from build123d import *

# Parameters (mm, degrees)
F1_DEPTH  = 12
F2_R      = 8
F3_DEPTH  = 12
F4_R      = 26
F5_DEPTH  = 46
F6_R      = 15
F7_DEPTH  = 12
F8_R      = 10
F9_DEPTH  = 34
F10_R     = 30
F10_R_2   = 26
F11_DEPTH = 12
F13_DEPTH = 46
F14_W     = 44.7685575615
F14_H     = 8
F15_DEPTH = 46
F17_DEPTH = 25


with BuildPart() as f1:
    # F0 (on Top) → F1 (new body)
    with BuildSketch(Plane.XY):
        with BuildLine():
            ThreePointArc((-54.3153104275, 3.1455838755), (-49.6290189265, -8.1681246235), (-38.3153104275, -12.8544161245))
            Line((-38.3153104275, -12.8544161245), (57.6846895725, -12.8544161245))
            ThreePointArc((57.6846895725, -12.8544161245), (68.9983980715, -8.1681246235), (73.6846895725, 3.1455838755))
            Line((73.6846895725, 3.1455838755), (73.6846895725, 36.1455838755))
            ThreePointArc((73.6846895725, 36.1455838755), (68.9983980715, 47.4592923745), (57.6846895725, 52.1455838755))
            Line((57.6846895725, 52.1455838755), (-38.3153104275, 52.1455838755))
            ThreePointArc((-38.3153104275, 52.1455838755), (-49.6290189265, 47.4592923745), (-54.3153104275, 36.1455838755))
            Line((-54.3153104275, 36.1455838755), (-54.3153104275, 3.1455838755))
        make_face()
    extrude(amount=F1_DEPTH)

    # F2 (on face) → F3 (cut)
    with BuildSketch(Plane.XY.offset(12)):
        with Locations((-38.7868596536, 37.2802639987)):
            Circle(F2_R)
        with Locations((-38.7868596536, 4.2802639987)):
            Circle(F2_R)
        with Locations((57.2131403464, 4.2802639987)):
            Circle(F2_R)
        with Locations((57.2131403464, 37.2802639987)):
            Circle(F2_R)
    extrude(amount=-F3_DEPTH, mode=Mode.SUBTRACT)

    # F4 (on face) → F5 (join)
    with BuildSketch(Plane.XY.offset(12)):
        with Locations((9.6846895725, 19.6455838755)):
            Circle(F4_R)
    extrude(amount=F5_DEPTH)

    # F6 (on face) → F7 (cut)
    with BuildSketch(Plane.XY.offset(58)):
        with Locations((9.6846895725, 19.6455838755)):
            Circle(F6_R)
    extrude(amount=-F7_DEPTH, mode=Mode.SUBTRACT)

    # F8 (on face) → F9 (cut)
    with BuildSketch(Plane.XY.offset(46)):
        with Locations((9.6846895725, 19.6455838755)):
            Circle(F8_R)
    extrude(amount=-F9_DEPTH, mode=Mode.SUBTRACT)

    # F10 (on face) → F11 (join)
    with BuildSketch(Plane.XY.offset(58)):
        with Locations((9.6846895725, 19.6455838755)):
            Circle(F10_R)
        with Locations((9.6846895725, 19.6455838755)):
            Circle(F10_R_2, mode=Mode.SUBTRACT)
    extrude(amount=-F11_DEPTH)

    # F12 (on face) → F13 (cut)
    with BuildSketch(Plane.XY.offset(58)):
        with BuildLine():
            Line((-9.546752866, -3.3794377691), (-9.546752866, 42.6706055201))
            ThreePointArc((-9.546752866, 42.6706055201), (-20.3153104275, 19.6455838755), (-9.546752866, -3.3794377691))
        make_face()
    extrude(amount=-F13_DEPTH, mode=Mode.SUBTRACT)

    # F14 (on face) → F15 (join)
    with BuildSketch(Plane.XY.offset(12)):
        with Locations((-31.9310316467, 19.6455838755)):
            Rectangle(F14_W, F14_H)
    extrude(amount=F15_DEPTH)

    # F16 (on face) → F17 (cut)
    with BuildSketch(Plane.XZ.offset(-15.6455838755)):
        Polygon((-54.3153104275, 12), (-9.546752866, 58), (-54.3153104275, 58), align=None)
    extrude(amount=-F17_DEPTH, mode=Mode.SUBTRACT)


solid = f1.part
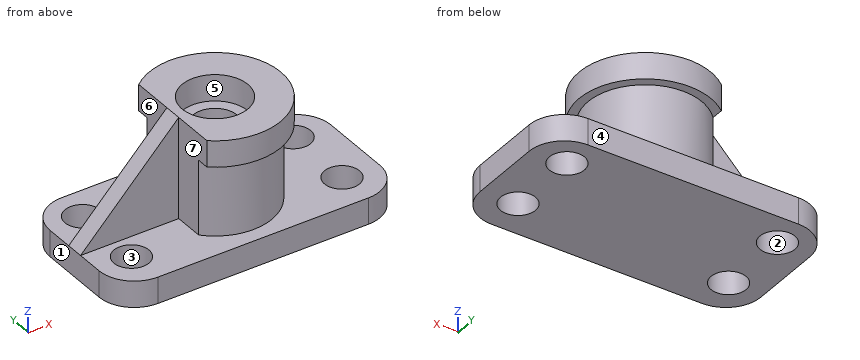
For this review, take the finished solid that the model builds, in its own axes (mm). Face numbers are marked on the shaded views. A direction names the side the tool comes from. Give positions to 0.01 mm unless a question says otherwise; leave off trailing zeros. Loops run counter-clockwise (first coordinate to the right, second up) from the corner with the lowest first, then second, coordinate; pieces in that order, holes last. Notation, with made-up numbers: M -30,-19 L -18,-19 A31 cw -18,13 Z; hole C -38,20 d8. An arc over 180 degrees is marked long. Put each result on its own line as item: value. Start each with the question number.
(1) Add section B-B, the plane z = 47.5. Write out the cut boundary in (x, y).
(2) Add section C-C, the plane x = -45. Write out the cut boundary in (y, z), then the cut area to 3 significant figures.
(3) The part is to be moulded in two halves that separate along Y. For the marked faces 1, 2, 3 and 4, say which applies: +Y half, -Y half, draft (parallel to the pull), parting line (faces both ways), or undercut.
(4) For pin 1 (21 mm diameter, centred on y = 11, z = 33, fed in from -X); pin 2 (3 mm diameter, centred on y = -2, z = 38.5, fed in from +X); pin 3 (21 mm diameter, centred on x = -38.79, y = 37.28, fed in from -Z); pin 4 (3 mm diameter, centred on y = 34, z = 48.5, fed in from -X), all flat-tipped, find the tip position at first contact; note any pin that passes through.
(5) Wall thickness on L1, parallel to X at y = 4, z = 11; L2, parallel to Z at x = 30.5, y = -0.5; L3, parallel to Z at x = 68.5, y = 15.5: over which ranges is each line inside the solid? List them lowest first.
(6) Add section D-D, the plane x = -13. Write out the cut boundary in (y, z).
(7) Machinability: for the marked faces 5, 6 and 7, which of the approach directions +Z, -Z, +X, -X, +Y, -Y give a long, thin tool a straight path to every point of the face, cutting with its end or side? Answer none if there is none.
(8) Add section A-A, the plane y = 11. Write out the cut boundary in (x, z).
Result:
1. outline: M -19.77,15.65 L -9.55,15.65 L -9.55,-3.38 A30 ccw long -9.55,42.67 L -9.55,23.65 L -19.77,23.65 Z; hole C 9.68,19.65 d30
2. outline: M -11.39,0 L -0.76,0 L -0.76,12 L -11.39,12 Z; M 9.32,0 L 32.24,0 L 32.24,12 L 23.65,12 L 23.65,21.57 L 15.65,21.57 L 15.65,12 L 9.32,12 Z; M 42.32,0 L 50.68,0 L 50.68,12 L 42.32,12 Z
2. area: 580 mm^2
3. face 1: draft
3. face 2: undercut
3. face 3: undercut
3. face 4: +Y half
4. pin 1: stops at x = -43.04
4. pin 2: stops at x = 26.12
4. pin 3: stops at z = 0
4. pin 4: stops at x = -9.55
5. L1: x = -54.32 to -46.78, -30.79 to 49.22, 65.21 to 73.68
5. L2: z = 0 to 12, 46 to 58
5. L3: z = 0 to 12
6. outline: M -12.85,0 L 52.15,0 L 52.15,12 L 23.65,12 L 23.65,54.45 L 15.65,54.45 L 15.65,12 L -12.85,12 Z
7. face 5: +Z
7. face 6: +Z, -X, +Y
7. face 7: +Z, -X, -Y
8. outline: M -54.32,0 L -43.13,0 L -43.13,12 L -54.32,12 Z; M -34.45,0 L 52.87,0 L 52.87,12 L 34.21,12 L 34.21,46 L 38.41,46 L 38.41,58 L 21.94,58 L 21.94,46 L 14.71,46 L 14.71,12 L 4.66,12 L 4.66,46 L -2.57,46 L -2.57,58 L -9.55,58 L -9.55,12 L -34.45,12 Z; M 61.55,0 L 73.68,0 L 73.68,12 L 61.55,12 Z
